Autodesk Inventor part; units mm, degrees
ref_plane "YZ Plane" through (0, 0, 0) normal (1, 0, 0) x (0, 1, 0)
ref_plane "XZ Plane" through (0, 0, 0) normal (0, 1, 0) x (-1, 0, 0)
ref_plane "XY Plane" through (0, 0, 0) normal (0, 0, 1) x (1, 0, 0)
sketch "Skizze1" plane through (0, 0, 0) normal (0, 1, 0) x (-1, 0, 0)
  line L0 (-27.5, 52.5) -> (27.5, 52.5)
  line L1 (27.5, 52.5) -> (27.5, -52.5)
  line L2 (27.5, -52.5) -> (-27.5, -52.5)
  line L3 (-27.5, -52.5) -> (-27.5, 52.5)
  line L4 (-27.5, 52.5) -> (27.5, -52.5) construction
  line L5 (27.5, 52.5) -> (-27.5, -52.5) construction
  point P0 (0, 0)
  dimension "d0" = 55
  dimension "d1" = 105
extrude "Extrusion1" add sketch "Skizze1" along normal blind 5
sketch "Skizze2" plane through (0, 5, 0) normal (0, 1, 0) x (1, 0, 0)
  line L0 (27.5, 52.5) -> (-27.5, 52.5)
  line L1 (-27.5, 52.5) -> (-27.5, -52.5)
  line L2 (-27.5, -52.5) -> (27.5, -52.5)
  line L3 (27.5, -52.5) -> (27.5, 52.5)
  line L4 (-27.5, -52.5) -> (27.5, -52.5)
  line L5 (27.5, -52.5) -> (27.5, -47.5)
  line L6 (27.5, -47.5) -> (-27.5, -47.5)
  line L7 (-27.5, -47.5) -> (-27.5, -52.5)
  line L8 (27.5, -47.5) -> (22.5, -47.5)
  line L9 (22.5, -47.5) -> (22.5, 52.5)
  line L10 (22.5, 52.5) -> (27.5, 52.5)
  line L11 (27.5, 52.5) -> (27.5, -47.5)
  line L12 (22.5, 52.5) -> (-27.5, 52.5)
  line L13 (-27.5, 52.5) -> (-27.5, 47.5)
  line L14 (-27.5, 47.5) -> (22.5, 47.5)
  line L15 (22.5, 47.5) -> (22.5, 52.5)
  point P0 (0, 0)
  dimension "d4" = 5
  dimension "d5" = 5
  dimension "d6" = 5
extrude "Extrusion2" add sketch "Skizze2" along normal blind 25 contours L3 L6 L9 L0 | L9 L14 L1 L0 | L3 L2 L1 L6
sketch "Skizze3" plane through (27.5, 0, -52.5) normal (0, 0, -1) x (-1, 0, 0)
  line L0 (0, 0) -> (55, 0)
  line L1 (55, 0) -> (55, 30)
  line L2 (0, 30) -> (55, 30)
  line L3 (0, 0) -> (0, 30)
  line L4 (55, 30) -> (0, 30)
  line L5 (0, 30) -> (0, 25)
  line L6 (0, 25) -> (55, 25)
  line L7 (55, 25) -> (55, 30)
  point P0 (27.5, 0)
  dimension "d9" = 5
extrude "Extrusion3" add sketch "Skizze3" along normal blind 20 contours L3 L2 L1 L6
sketch "Skizze4" plane through (-27.5, 0, 52.5) normal (0, 0, 1) x (1, 0, 0)
  line L0 (0, 0) -> (55, 0)
  line L1 (55, 0) -> (55, 30)
  line L2 (0, 30) -> (55, 30)
  line L3 (0, 0) -> (0, 30)
  line L4 (55, 25) -> (0, 25)
  line L5 (0, 30) -> (55, 30)
  line L6 (55, 30) -> (55, 25)
  line L7 (55, 25) -> (0, 25)
  line L8 (0, 25) -> (0, 30)
  point P0 (27.5, 0)
  dimension "d12" = 5
extrude "Extrusion4" add sketch "Skizze4" along normal blind 20 contours L3 L2 L1 L4
sketch "Skizze5" plane through (0, 30, 0) normal (0, 1, 0) x (1, 0, 0)
  line L0 (-27.5, -47.5) -> (-27.5, -72.5)
  line L1 (27.5, -72.5) -> (-27.5, -72.5)
  line L2 (27.5, 72.5) -> (27.5, -72.5)
  line L3 (-27.5, 72.5) -> (27.5, 72.5)
  line L4 (-27.5, 47.5) -> (-27.5, 72.5)
  line L5 (-27.5, 47.5) -> (22.5, 47.5)
  line L6 (22.5, 47.5) -> (22.5, -47.5)
  line L7 (22.5, -47.5) -> (-27.5, -47.5)
  line L8 (0, 72.5) -> (0, 62.5)
  circle A0 centre (0, 62.5) radius 3.1
  line L9 (0, -72.5) -> (0, -62.5)
  circle A1 centre (0, -62.5) radius 3.1
  point P0 (0, 0)
  dimension "d15" = 10
  dimension "d16" = 6.2
  dimension "d17" = 10
  dimension "d18" = 6.2
extrude "Extrusion5" cut sketch "Skizze5" against normal blind 20 contours A1 | A0
sketch "Skizze6" plane through (0, 30, 0) normal (0, 1, 0) x (1, 0, 0)
  circle A0 centre (0, 62.5) radius 3.1
  circle A1 centre (0, -62.5) radius 3.1
  line L0 (-27.5, -47.5) -> (-27.5, -72.5)
  line L1 (27.5, -72.5) -> (-27.5, -72.5)
  line L2 (27.5, 72.5) -> (27.5, -72.5)
  line L3 (-27.5, 72.5) -> (27.5, 72.5)
  line L4 (-27.5, 47.5) -> (-27.5, 72.5)
  line L5 (-27.5, 47.5) -> (22.5, 47.5)
  line L6 (22.5, 47.5) -> (22.5, -47.5)
  line L7 (22.5, -47.5) -> (-27.5, -47.5)
  line L8 (22.5, -47.5) -> (27.5, -47.5)
  line L9 (22.5, -47.5) -> (22.5, -42.5)
  line L10 (22.5, -42.5) -> (27.5, -42.5)
  line L11 (22.5, -42.5) -> (22.5, -7.5)
  line L12 (22.5, 47.5) -> (22.5, -47.5)
  line L13 (22.5, -7.5) -> (27.5, -7.5)
  point P0 (0, 0)
  dimension "d21" = 5
  dimension "d22" = 35
extrude "Extrusion6" cut sketch "Skizze6" against normal blind 20 contours L6 L13 L2 L10
properties part number "Hub"
The model under review builds one solid part; all positions refer to its coordinate system, in mm. A direction names the side the tool comes from. Give positions to 0.01 mm unless a question says otherwise; leave off trailing zeros. Loops run counter-clockwise (first coordinate to the right, second up) from the corner with the lowest first, then second, coordinate; pieces in that order, holes last. Notation, with made-up numbers: (51.25, 62) -> (92.25, 62) arc R27 cw to (92.25, 86) -> close; hole circle Ø6 at (62, 81). An arc over 180 degrees is marked (long way). Put each result on its own line as item: value. Start each with the question number.
1. We need section B-B on x = 18.5. State the section outline as (y, z) points.
2. Wall thickness on probe 1 along Z at (x, y) = (0, 28.95); probe 2 along Z at (x, y) = (4, 25.5); probe 3 along X at (y, z) = (28.25, 62.5): over which ranges is each line inside the solid? List them lowest first.
3. Clearance check with flat-ended pins moving along their axes: P1, Ø10, axis at x = 0, z = -62.5, coming from the -Y side; P2, Ø22, axis at x = 7.5, z = -59.5, coming from the -Y side; P3, Ø1, axis at x = -9.5, z = -22, coming from the +Y side; P4, Ø2, axis at x = 21.5, y = 13, coming from the -Z side. State where each tip first meets the part, or that it passes through.
4. We need section A-A on z = 62.5. State the section outline as (x, y) points.
5. Mouldability with a two-part tool opening along Z and no side actions: class faces 6 (the face through (0, 25, -58)), 7 (the face through (-2, 17, 47.5)), 8 (the face through (0, 28, 72.5)) as released by +Z, released by -Z, zero draft, split by the parting line, or undercut.
6. We need section C-C on y = 21. State the section outline as (x, z) points, then the cut area to 3 significant figures.
7. We need section D-D on x = 0. State the section outline as (y, z) points.
8. For faces 1 (the face through (-3, 17, -47.5)), 2 (the face through (25, 10, 25)), 3 (the face through (0, 12, -52.5)), 4 (the face through (0, 12, 52.5)), 5 (the face through (6, 30, -51)), list the 3-axis set-ups (+Z, -Z, +X, -X, +Y, -Y) from which the entire face can be reached by the end or side of a thin tool; tool diameter is ignored.
Determined:
1. outline: (0, -52.5) -> (25, -52.5) -> (25, -72.5) -> (30, -72.5) -> (30, -47.5) -> (5, -47.5) -> (5, 47.5) -> (30, 47.5) -> (30, 72.5) -> (25, 72.5) -> (25, 52.5) -> (0, 52.5) -> close
2. probe 1: -72.5 to -65.6, -59.4 to -47.5, 47.5 to 59.4, 65.6 to 72.5
2. probe 2: -72.5 to -47.5, 47.5 to 72.5
2. probe 3: -27.5 to -3.1, 3.1 to 27.5
3. P1: y = 25
3. P2: y = 0
3. P3: y = 5
3. P4: z = -52.5
4. outline: (-27.5, 25) -> (-3.1, 25) -> (-3.1, 30) -> (-27.5, 30) -> close; (3.1, 25) -> (27.5, 25) -> (27.5, 30) -> (3.1, 30) -> close
5. face 6: zero draft
5. face 7: undercut
5. face 8: released by +Z
6. outline: (-27.5, -52.5) -> (27.5, -52.5) -> (27.5, 7.5) -> (22.5, 7.5) -> (22.5, -47.5) -> (-27.5, -47.5) -> close; (-27.5, 47.5) -> (22.5, 47.5) -> (22.5, 42.5) -> (27.5, 42.5) -> (27.5, 52.5) -> (-27.5, 52.5) -> close
6. area: 850 mm^2
7. outline: (0, -52.5) -> (25, -52.5) -> (25, -59.4) -> (30, -59.4) -> (30, -47.5) -> (5, -47.5) -> (5, 47.5) -> (30, 47.5) -> (30, 59.4) -> (25, 59.4) -> (25, 52.5) -> (0, 52.5) -> close; (25, -72.5) -> (30, -72.5) -> (30, -65.6) -> (25, -65.6) -> close; (25, 65.6) -> (30, 65.6) -> (30, 72.5) -> (25, 72.5) -> close
8. face 1: -X, +Y
8. face 2: +X, -X, +Y
8. face 3: -Z, +X, -X, -Y
8. face 4: +Z, +X, -X, -Y
8. face 5: +Z, -Z, +X, -X, +Y
